Verification items for the finished model (mm, model axes). Coordinates: 2 decimals unless noted, no trailing zeros. Loops run counter-clockwise (first coordinate to the right, second up) from the corner with the lowest first, then second, coordinate; pieces in that order, holes last. Notation, with made-up numbers: (53, 83.25) -> (87, 83.25) arc R18 ccw to (87, 117.25) -> close; hole circle Ø7 at (66.5, 11). An arc over 180 degrees is marked (long way). Answer as a JSON object with one key per item and string values. Group by question number.
Q1. Release check for a two-part mould opening along Z. For faces 1 (the flat face through (0, 0, -8)), 2 (the cylindrical face through (3.365, -15.065, 0.091)), 3 (the cylindrical face through (2.763, 8.767, -16.856)) record: released by +Z, released by -Z, zero draft, split by the parting line, or undercut.
Q2. Cross-section at B-B on x = 1. Record the boundary of the cut face in (y, z).
Q3. Cross-section at C-C on y = 0. Give the number of separate pieces and of enclosed holes in the cut face, and give its area (3 significant figures).
Q4. Gauge pin test, flat ends, axial feed: pin 1 Ø3.5 at (y, z) = (13, 0) entering from +X; pin 2 Ø3 at (x, y) = (5, -10) entering from -Z; pin 3 Ø5.5 at (y, z) = (-13, 0) entering from +X; pin 4 Ø1.5 at (x, z) = (2, 7.5) entering from -Y. Record the tip position at first contact, or that the pin passes through.
Q5. Cross-section at A-A on z = 0. Record the boundary of the cut face in (x, y).
Q6. Cross-section at D-D on x = 4.5. Record the boundary of the cut face in (y, z), and give its area (3 significant figures).
Q7. Scan lines: L1, parallel to Z at x = 1.5, y = 3; L2, parallel to Y at x = 5.75, z = 6.5; L3, parallel to Z at x = 5.5, y = 1.5. Record each from-to range of solid material in increasing order.
Autodesk Inventor part; units mm, degrees
ref_plane "at1_dgb_st_XY" through (0, 0, 0) normal (1, 0, 0) x (0, 0, -1)
ref_plane "at1_dgb_st_YZ" through (0, 0, 0) normal (0, 0, -1) x (0, 1, 0)
ref_plane "at1_dgb_st_ZX" through (0, 0, 0) normal (0, 1, 0) x (1, 0, 0)
sketch "Sketch_10" plane through (0, 0, 0) normal (0, 0, 1) x (1, 0, 0)
  line L0 (6.65, 0) -> (0, 0)
  line L1 (0, 0) -> (0, 19)
  line L2 (0, 19) -> (5.45, 19)
  line L3 (5.45, 19) -> (6.65, 17.8)
  line L4 (6.65, 17.8) -> (6.65, 0)
  line L5 (6.65, 0) -> (0, 0)
revolve "Revolution1" add sketch "Sketch_10" angle 360 about axis through (6.65, 0, 0) along (1, 0, 0)
sketch "Sketch_11" plane through (0, 0, 0) normal (0, 0, 1) x (1, 0, 0)
  line L0 (6.65, 0) -> (0, 0)
  line L1 (0, 0) -> (0, 7.6)
  line L2 (0, 7.6) -> (6.65, 9.728)
  line L3 (6.65, 9.728) -> (6.65, 0)
  line L4 (6.65, 0) -> (0, 0)
revolve "Revolution2" cut sketch "Sketch_11" angle 360 about axis through (6.65, 0, 0) along (1, 0, 0)
sketch "Sketch_12" plane through (0, 0, 0) normal (0, 0, 1) x (1, 0, 0)
  line L0 (6.65, 13) -> (0, 13)
  line L1 (0, 13) -> (0, 15.5)
  line L2 (0, 15.5) -> (0.433, 15.067)
  line L3 (0.433, 15.067) -> (6.217, 15.067)
  line L4 (6.217, 15.067) -> (6.65, 15.5)
  line L5 (6.65, 15.5) -> (6.65, 13)
  line L6 (6.65, 13) -> (0, 13)
revolve "Revolution3" cut sketch "Sketch_12" angle 360 about axis through (6.65, 13, 0) along (1, 0, 0)
thread "Thread1"
pattern_linear "Rectangular Pattern1" count 2 spacing 18.3848 along (0, -0.7071, 0.7071) count 2 spacing 18.3848 along (0, -0.7071, -0.7071) of "Revolution3"
ref_plane "at1_dgb_st_XY" through (0, 0, 0) normal (1, 0, 0) x (0, 0, -1)
ref_plane "at1_dgb_st_YZ" through (0, 0, 0) normal (0, 0, -1) x (0, 1, 0)
ref_plane "at1_dgb_st_ZX" through (0, 0, 0) normal (0, 1, 0) x (1, 0, 0)
ref_plane "at_gew_XY" through (15, 0, 0) normal (1, 0, 0) x (0, 0, -1)
ref_plane "at_gew_YZ" through (15, 0, 0) normal (0, 0, -1) x (0, 1, 0)
ref_plane "at_gew_ZX" through (15, 0, 0) normal (0, 1, 0) x (1, 0, 0)
ref_plane "it_schrschei_XY" through (7.5, 0, 0) normal (1, 0, 0) x (0, 0, -1)
ref_plane "it_schrschei_YZ" through (7.5, 0, 0) normal (0, 0, -1) x (0, 1, 0)
ref_plane "it_schrschei_ZX" through (7.5, 0, 0) normal (0, 1, 0) x (1, 0, 0)
properties part number "61581400_2"
Computed values:
{
 "1": {"face 1": "zero draft", "face 2": "undercut", "face 3": "split by the parting line"},
 "2": {"outline": "circle Ø38 at (0, 0); hole circle Ø4.13 at (-13, 0); hole circle Ø15.84 at (0, 0); hole circle Ø4.13 at (0, -13); hole circle Ø4.13 at (0, 13); hole circle Ø4.13 at (13, 0)"},
 "3": {"separate pieces": "4", "enclosed holes": "0", "area": "80.3 mm²"},
 "4": {"pin 1": "passes through", "pin 2": "stops at z = -16.99", "pin 3": "stops at x = 6.65", "pin 4": "stops at y = -17.76"},
 "5": {"outline": "(0, -19) -> (5.45, -19) -> (6.65, -17.8) -> (6.65, -15.5) -> (6.22, -15.07) -> (0.43, -15.07) -> (0, -15.5) -> close; (0, -10.5) -> (0.43, -10.93) -> (6.22, -10.93) -> (6.65, -10.5) -> (6.65, -9.73) -> (0, -7.6) -> close; (0, 7.6) -> (6.65, 9.73) -> (6.65, 10.5) -> (6.22, 10.93) -> (0.43, 10.93) -> (0, 10.5) -> close; (0, 15.5) -> (0.43, 15.07) -> (6.22, 15.07) -> (6.65, 15.5) -> (6.65, 17.8) -> (5.45, 19) -> (0, 19) -> close"},
 "6": {"outline": "circle Ø38 at (0, 0); hole circle Ø4.13 at (-13, 0); hole circle Ø18.08 at (0, 0); hole circle Ø4.13 at (0, -13); hole circle Ø4.13 at (0, 13); hole circle Ø4.13 at (13, 0)", "area": "824 mm²"},
 "7": {"L1": "z = -18.76 to -7.5, 7.5 to 18.76", "L2": "y = -17.53 to -6.85, 6.85 to 17.53", "L3": "z = -18.89 to -14.42, -11.58 to -9.24, 9.24 to 11.58, 14.42 to 18.89"}
}
